Autodesk Inventor part; units mm, degrees
ref_plane "YZ Plane" through (0, 0, 0) normal (1, 0, 0) x (0, 1, 0)
ref_plane "XZ Plane" through (0, 0, 0) normal (0, 1, 0) x (-1, 0, 0)
ref_plane "XY Plane" through (0, 0, 0) normal (0, 0, 1) x (1, 0, 0)
sketch "Sketch8" plane through (0, 0, 0) normal (0, 1, 0) x (-1, 0, 0)
  line L0 (83, 40) -> (-83, 40)
  line L1 (-83, 40) -> (-83, -40)
  line L2 (-83, -40) -> (83, -40)
  line L3 (83, -40) -> (83, 40)
  line L4 (83, 40) -> (-83, -40) construction
  line L5 (-83, 40) -> (83, -40) construction
  point P0 (0, 0)
  dimension "d28" = 80
  dimension "d29" = 166
extrude "Extrusion8" add sketch "Sketch8" against normal blind 8
sketch "Sketch11" plane through (0, 0, 0) normal (0, 1, 0) x (1, 0, 0)
  line L0 (83, 40) -> (-83, 40)
  line L1 (-83, -40) -> (83, -40)
  line L2 (-83, 40) -> (-83, -40)
  line L3 (83, -40) -> (83, 40)
  line L4 (-31.038, -40) -> (-9.602, 40)
  line L5 (-9.602, 40) -> (-17.8842, 40)
  line L6 (-75, 40) -> (75, 40)
  line L7 (-17.8842, 40) -> (-39.3202, -40)
  line L8 (-39.3202, -40) -> (-31.038, -40)
  line L9 (-31.038, -40) -> (-31.038, 40) construction
  line L10 (0, -40) -> (0, 40) construction
  line L11 (9.602, -40) -> (31.038, 40)
  line L12 (31.038, 40) -> (39.3202, 40)
  line L13 (39.3202, 40) -> (17.8842, -40)
  line L14 (17.8842, -40) -> (9.602, -40)
  point P0 (0, 0)
  point P1 (0, -40)
  point P2 (0, -40)
  point P3 (-20.32, 0)
  point P4 (0, 0)
  point P5 (20.32, 0)
  point P6 (39.3202, 40)
  point P7 (31.038, 40)
  point P8 (-17.8842, 40)
  dimension "d39" = -15
  dimension "d40" = 8
  dimension "d42" = 8
  dimension "d44" = 20.32
  dimension "d45" = 20.32
extrude "Extrusion11" add sketch "Sketch11" along normal blind 104.1375 contours L13 L1 L11 L0 | L4 L1 L7 L0
sketch "Sketch12" plane through (0, 0, 0) normal (0, 1, 0) x (1, 0, 0)
  line L0 (31.038, 40) -> (-9.602, 40)
  line L1 (31.038, 40) -> (9.602, -40)
  line L2 (-31.038, -40) -> (9.602, -40)
  line L3 (-31.038, -40) -> (-9.602, 40)
  line L4 (-9.602, 40) -> (31.038, 40)
  line L5 (31.038, 40) -> (9.602, -40)
  line L6 (9.602, -40) -> (-31.038, -40)
  line L7 (-9.602, 40) -> (-31.038, -40)
  line L8 (-31.038, -40) -> (-9.602, 40)
  point P0 (0, 0)
extrude "Extrusion12" add sketch "Sketch12" along normal blind 20
sketch "Sketch15" plane through (-39.3202, 0, 40) normal (-0.9659, 0, -0.2588) x (-0.2588, 0, 0.9659)
  line L0 (-82.8221, 104.1375) -> (0, 104.1375)
  line L1 (0, 0) -> (0, 104.1375)
  line L2 (-82.8221, 0) -> (-82.8221, 104.1375)
  line L3 (-2.1436, 20) -> (-84.9657, 20)
  line L4 (-82.8221, 40) -> (0, 40) construction
  line L5 (-67.8221, 40) -> (-67.8221, 104.1375) construction
  point P0 (-48.8138, 0)
  point P1 (-82.8221, 52.0688)
  point P2 (-47.8221, 40)
  point P3 (-27.8221, 40)
  point P4 (-67.8221, 60)
  point P5 (-47.8221, 60)
  point P6 (-27.8221, 60)
  point P7 (-67.8221, 80)
  point P8 (-47.8221, 80)
  point P9 (-27.8221, 80)
  dimension "d64" = 15
  dimension "d74" = 20
  dimension "d77" = 20
  dimension "d90" = 20
hole "HoleForLeftSideOf2x4" at (-21.7665, 40, -25.5111) at (-26.9429, 40, -6.1926) at (-32.1193, 40, 13.1259) at (-26.9429, 60, -6.1926) at (-21.7665, 60, -25.5111) at (-32.1193, 60, 13.1259) at (-32.1193, 80, 13.1259) at (-26.9429, 80, -6.1926) at (-21.7665, 80, -25.5111) direction (0.9659, 0, 0.2588) diameter 4.496 depth 8 countersink diameter 8.433 countersink angle 82
sketch "Sketch16" plane through (39.3202, 0, -40) normal (0.9659, 0, 0.2588) x (0.2588, 0, -0.9659)
  line L0 (-82.8221, 104.1375) -> (0, 104.1375)
  line L1 (0, 0) -> (0, 104.1375)
  line L2 (-82.8221, 0) -> (-82.8221, 104.1375)
  line L3 (-82.8221, 0) -> (-65.9689, 0)
  line L4 (-2.1436, 20) -> (-84.9657, 20)
  line L5 (-82.8221, 40) -> (0, 40) construction
  line L6 (-67.8221, 40) -> (-67.8221, 104.1375) construction
  point P0 (-48.8138, 0)
  point P1 (-47.8221, 40)
  point P2 (-27.8221, 40)
  point P3 (-67.8221, 60)
  point P4 (-47.8221, 60)
  point P5 (-27.8221, 60)
  point P6 (-67.8221, 80)
  point P7 (-47.8221, 80)
  point P8 (-27.8221, 80)
  dimension "d80" = 20
  dimension "d81" = 15
  dimension "d84" = 20
  dimension "d87" = 20
hole "HolesForRightSideOf2x4" at (26.9429, 40, 6.1926) at (32.1193, 40, -13.1259) at (21.7665, 60, 25.5111) at (26.9429, 60, 6.1926) at (32.1193, 60, -13.1259) at (21.7665, 80, 25.5111) at (26.9429, 80, 6.1926) at (32.1193, 80, -13.1259) at (21.7665, 40, 25.5111) direction (-0.9659, 0, -0.2588) diameter 4.496 depth 8 countersink diameter 8.433 countersink angle 82
equation "\"d28\" = widthOfBracket"
equation "\"d30\" = wallThickness"
equation "\"d39\" = azimuth"
equation "\"d40\" = wallThickness"
equation "\"d42\" = wallThickness"
equation "\"d46\" = twoByFourDepth + baseBelowTwoByFour"
equation "\"d49\" = baseBelowTwoByFour"
equation "\"wallThickness\" = 8"
equation "\"widthOfBracket\" = 80"
equation "\"twoByFourWidth\" = 40.64"
equation "\"twoByFourDepth\" = 84.1375"
equation "\"azimuth\" = -15deg"
equation "\"elevation\" = 20deg"
equation "\"baseBelowTwoByFour\" = 20"
equation "\"centerForTwoHoles\" = 0.25 * diagonalLine"
equation "\"depthOfExtrusionForMatingToLowerHalf\" = 12.5"
equation "\"depthForWasherForMatingToCase\" = 14"
properties part number "pvcBracketUpperPortion" material "PC/ABS Plastic"
Could you check a few things on this model? Use its own coordinates, in mm. A direction names the side the tool comes from. Give positions to 0.01 mm unless a question says otherwise; leave off trailing zeros. Loops run counter-clockwise (first coordinate to the right, second up) from the corner with the lowest first, then second, coordinate; pieces in that order, holes last. Notation, with made-up numbers: (19, 82.25) -> (49, 82.25) arc R12 ccw to (49, 90.25) -> close; hole circle Ø5 at (53, 76). An arc over 180 degrees is marked (long way). Put each result on its own line as item: value.
(1) Imagine slicing it at D-D on x = -61. Write out the boundary of the cut face in (y, z).
Computed:
outline: (-8, -40) -> (0, -40) -> (0, 40) -> (-8, 40) -> close
(2) Imagine slicing it at A-A on y = 68.5. Write out the boundary of the cut face in (x, z), plus the area to 3 significant figures.
Computed:
outline: (-39.32, 40) -> (-17.88, -40) -> (-9.6, -40) -> (-31.04, 40) -> close; (9.6, 40) -> (31.04, -40) -> (39.32, -40) -> (17.88, 40) -> close
area: 1,330 mm^2
(3) Imagine slicing it at B-B on z = 34. Write out the boundary of the cut face in (x, y), plus the area to 3 significant figures.
Computed:
outline: (-83, -8) -> (83, -8) -> (83, 0) -> (19.49, 0) -> (19.49, 104.14) -> (11.21, 104.14) -> (11.21, 20) -> (-29.43, 20) -> (-29.43, 104.14) -> (-37.71, 104.14) -> (-37.71, 0) -> (-83, 0) -> close
area: 3,870 mm^2
(4) Thinking about a two-plate mould opening in X: for faces 4 (the face through (-27.05, 37.77, 14.18)), 5 (the face through (-83, -4, -1)), 6 (the face through (1, -8, 1)), 7 (the face through (27.05, 37.77, -14.18)), which applies, pulls with the +X half, pulls with the -X half, needs draft (parallel to the pull), parting line crosses it, or undercut?
Computed:
face 4: undercut
face 5: pulls with the -X half
face 6: needs draft
face 7: undercut
(5) For faces 1 (the face through (28.752, 51.34, -0.56)), 2 (the face through (20.17, 61.48, 0.56)), 3 (the face through (21.87, 37.77, 5.14)), which set-ups out of +Z, -Z, +X, -X, +Y, -Y let a thin tool reach every point of the face, with its end or its side?
Computed:
face 1: +Z, +X, +Y
face 2: -Z, +Y
face 3: none
(6) Imagine slicing it at C-C on x = 7. Write out the boundary of the cut face in (y, z).
Computed:
outline: (-8, -40) -> (20, -40) -> (20, 40) -> (-8, 40) -> close
(7) I'm going to push flat-ended pins straight in: pin 1 Ø1 at (y, z) = (15, 22.5) entering from -X; pin 2 Ø5 at (y, z) = (49.5, 27.5) entering from -X; pin 3 Ø2 at (y, z) = (79.5, -30.5) entering from +X. Where does each tip first touch, or does it pass through?
Computed:
pin 1: x = -34.77
pin 2: x = -36.64
pin 3: x = 37.04
(8) Please list where these lines run through material, in increasing order: probe 1 along Y at (x, z) = (-38.5, -10); probe 2 along Y at (x, z) = (-16, 14.5); probe 3 along X at (y, z) = (25.5, -36). Write a range as [from, to].
Computed:
probe 1: [-8, 0]
probe 2: [-8, 20]
probe 3: [-18.96, -10.67], [29.97, 38.25]
